```python
from build123d import *

# Parameters (mm, degrees)
SKETCH1_W                    = 79.375
SKETCH1_H                    = 381
BASE_FLANGE1_DEPTH           = 3.175
EDGE_FLANGE1_STRIP_W         = 19.05
EDGE_FLANGE1_STRIP_H         = 3.175
EDGE_FLANGE1_STRIP_CUT_DEPTH = 381
EDGE_FLANGE1_DEPTH           = 381
EDGE_FLANGE2_STRIP_W         = 19.05
EDGE_FLANGE2_STRIP_H         = 3.175
EDGE_FLANGE2_STRIP_CUT_DEPTH = 381
EDGE_FLANGE2_DEPTH           = 381
EDGE_FLANGE3_STRIP_W         = 19.05
EDGE_FLANGE3_STRIP_H         = 3.175
EDGE_FLANGE3_STRIP_CUT_DEPTH = 381
EDGE_FLANGE3_DEPTH           = 381
SKETCH24_W                   = 50.8
SKETCH24_H                   = 31.496
TAB3_DEPTH                   = 3.175
SKETCH27_W                   = 76.2
SKETCH27_H                   = 31.496
TAB4_DEPTH                   = 3.175
SKETCH30_R                   = 1.5875
CUT_EXTRUDE2_DEPTH           = 466.600516135
SKETCH31_R                   = 1.5875
CUT_EXTRUDE3_DEPTH           = 466.600516135


# Sheet-metal steps are written as plain solids
with BuildPart() as part:
    # Sketch1 → Base-Flange1 (new body)
    with BuildSketch(Plane(origin=(0, 0, 0), x_dir=(1, 0, 0), z_dir=(0, 1, 0))):
        with Locations((39.6875, 190.5)):
            Rectangle(SKETCH1_W, SKETCH1_H)
    extrude(amount=-BASE_FLANGE1_DEPTH)

    # Edge-Flange1 strip (across the edge) → Edge-Flange1 strip cut (cut)
    with BuildSketch(Plane.XY.offset(-381)):
        with Locations((-6.35, -1.5875)):
            Rectangle(EDGE_FLANGE1_STRIP_W, EDGE_FLANGE1_STRIP_H)
    extrude(amount=EDGE_FLANGE1_STRIP_CUT_DEPTH, mode=Mode.SUBTRACT)

    # Edge-Flange1 section (across the edge) → Edge-Flange1 (add)
    with BuildSketch(Plane.XY.offset(-381)):
        with BuildLine():
            Line((-3.175, 3.175), (-3.175, 34.925))
            Line((-3.175, 34.925), (0, 34.925))
            Line((0, 34.925), (0, 3.175))
            ThreePointArc((0, 3.175), (0.92993597, 0.92993597), (3.175, 0))
            Line((3.175, 0), (3.175, -3.175))
            ThreePointArc((3.175, -3.175), (-1.315128061, -1.315128061), (-3.175, 3.175))
        make_face()
    extrude(amount=EDGE_FLANGE1_DEPTH)

    # Edge-Flange2 strip (across the edge) → Edge-Flange2 strip cut (cut)
    with BuildSketch(Plane(origin=(0, 34.925, -381), x_dir=(0, -1, 0), z_dir=(0, 0, 1))):
        with Locations((-6.35, -1.5875)):
            Rectangle(EDGE_FLANGE2_STRIP_W, EDGE_FLANGE2_STRIP_H)
    extrude(amount=EDGE_FLANGE2_STRIP_CUT_DEPTH, mode=Mode.SUBTRACT)

    # Edge-Flange2 section (across the edge) → Edge-Flange2 (add)
    with BuildSketch(Plane(origin=(0, 34.925, -381), x_dir=(0, -1, 0), z_dir=(0, 0, 1))):
        with BuildLine():
            Line((-3.175, 3.175), (-3.175, 76.2))
            Line((-3.175, 76.2), (0, 76.2))
            Line((0, 76.2), (0, 3.175))
            ThreePointArc((0, 3.175), (0.92993597, 0.92993597), (3.175, 0))
            Line((3.175, 0), (3.175, -3.175))
            ThreePointArc((3.175, -3.175), (-1.315128061, -1.315128061), (-3.175, 3.175))
        make_face()
    extrude(amount=EDGE_FLANGE2_DEPTH)

    # Edge-Flange3 strip (across the edge) → Edge-Flange3 strip cut (cut)
    with BuildSketch(Plane(origin=(76.2, 34.925, -381), x_dir=(-1, 0, 0), z_dir=(0, 0, 1))):
        with Locations((-6.35, -1.5875)):
            Rectangle(EDGE_FLANGE3_STRIP_W, EDGE_FLANGE3_STRIP_H)
    extrude(amount=EDGE_FLANGE3_STRIP_CUT_DEPTH, mode=Mode.SUBTRACT)

    # Edge-Flange3 section (across the edge) → Edge-Flange3 (add)
    with BuildSketch(Plane(origin=(76.2, 34.925, -381), x_dir=(-1, 0, 0), z_dir=(0, 0, 1))):
        with BuildLine():
            Line((-3.175, 3.175), (-3.175, 34.671))
            Line((-3.175, 34.671), (0, 34.671))
            Line((0, 34.671), (0, 3.175))
            ThreePointArc((0, 3.175), (0.92993597, 0.92993597), (3.175, 0))
            Line((3.175, 0), (3.175, -3.175))
            ThreePointArc((3.175, -3.175), (-1.315128061, -1.315128061), (-3.175, 3.175))
        make_face()
    extrude(amount=EDGE_FLANGE3_DEPTH)

    # Sketch24 → Tab3 (add)
    with BuildSketch(Plane.ZY.offset(-76.2)):
        with Locations((25.4, 16.002)):
            Rectangle(SKETCH24_W, SKETCH24_H)
    extrude(amount=-TAB3_DEPTH)

    # Sketch27 → Tab4 (add)
    with BuildSketch(Plane.ZY.offset(-76.2)):
        with Locations((-419.1, 16.002)):
            Rectangle(SKETCH27_W, SKETCH27_H)
    extrude(amount=-TAB4_DEPTH)

    # Sketch30 → Cut-Extrude2 (cut, through all)
    with BuildSketch(Plane.ZY.offset(-76.2)):
        with Locations(Location((10.16, 25.527, 0), (0, 0, 270))):
            Circle(SKETCH30_R)
        with Locations(Location((41.91, 25.527, 0), (0, 0, 270))):
            Circle(SKETCH30_R)
        with Locations(Location((41.91, 6.477, 0), (0, 0, 270))):
            Circle(SKETCH30_R)
        with Locations(Location((10.16, 6.477, 0), (0, 0, 270))):
            Circle(SKETCH30_R)
    extrude(amount=-CUT_EXTRUDE2_DEPTH, mode=Mode.SUBTRACT)

    # Sketch31 → Cut-Extrude3 (cut, through all)
    with BuildSketch(Plane.ZY.offset(-76.2)):
        with Locations(Location((-447.675, 25.527, 0), (0, 0, 270))):
            Circle(SKETCH31_R)
        with Locations(Location((-447.675, 6.477, 0), (0, 0, 270))):
            Circle(SKETCH31_R)
    extrude(amount=-CUT_EXTRUDE3_DEPTH, mode=Mode.SUBTRACT)


solid = part.part
```
The model under review builds one solid part; all positions refer to its coordinate system, in mm. A direction names the side the tool comes from. Coordinates: 2 decimals unless noted, no trailing zeros. Order: outer loops, then holes, each group sorted by start corner. A loop starts at its lowest first (then second) coordinate and runs counter-clockwise, first axis right, second up. Notation, with made-up numbers: M -33,20 L -16,20 A19 ccw -16,34 Z; hole C 23,25 d9. An arc over 180 degrees is marked long. One line per question, with ' | ' between items.
(1) Insertion check: pin 1 (2.5 mm diameter, centred on x = 78.5, z = -403.5, fed in from +Y); pin 2 (1.9 mm diameter, centred on y = 25.527, z = 10.16, fed in from -X); pin 3 (10 mm diameter, centred on x = 22, y = 3, fed in from +Z). Each pin has a flat end and moves straight along its axis. Give the tip position at first contact, or say it passes through.
Geometry results:
pin 1: stops at y = 31.75 | pin 2: passes through | pin 3: stops at z = 0
(2) The part is to be moulded in two halves that separate along Y. For faces 1 (the face through (-3.175, 17, -193)), 2 (the face through (38, 38.1, -193)), 3 (the face through (41, -3.175, -193)), 4 (the face through (41, 0, -193)), say which applies: +Y half, -Y half, draft (parallel to the pull), parting line (faces both ways), or undercut.
Geometry results:
face 1: draft | face 2: +Y half | face 3: -Y half | face 4: undercut
(3) Add section C-C, the plane z = -225.5. Write out the cut boundary in (x, y) (3 decimals).
Geometry results:
outline: M -3.175,3.175 A6.35 ccw 3.175,-3.175 L 79.375,-3.175 L 79.375,0 L 3.175,0 A3.175 cw 0,3.175 L 0,31.75 A3.175 cw 3.175,34.925 L 73.025,34.925 A3.175 cw 76.2,31.75 L 76.2,0.254 L 79.375,0.254 L 79.375,31.75 A6.35 ccw 73.025,38.1 L 3.175,38.1 A6.35 ccw -3.175,31.75 Z
(4) Machinability: for faces 5 (the face through (0, 18, -193)), 6 (the face through (79.375, 16, -207)), which of the approach directions +Z, -Z, +X, -X, +Y, -Y give a long, thin tool a straight path to every point of the face, cutting with its end or side? Answer none if there is none.
Geometry results:
face 5: +Z, -Z | face 6: +Z, -Z, +X, +Y, -Y
(5) For probe 1 along Y at (x, z) = (53, -266) (3 decimals); probe 2 along X at (y, z) = (22.5, -322) (3 decimals); probe 3 along Y at (x, z) = (77, 10), list the stretches that pass through material, from the lowest coordinate up. Write a range as from..to.
Geometry results:
probe 1: y = -3.175..0, 34.925..38.1 | probe 2: x = -3.175..0, 76.2..79.375 | probe 3: y = 0.25..4.9, 8.06..23.95, 27.11..31.75
(6) Add section A-A, the plane y = 19.5. Write out the cut boundary in (x, z) (3 decimals), then the cut area to 3 significant figures.
Geometry results:
outline: M -3.175,-381 L 0,-381 L 0,0 L -3.175,0 Z; M 76.2,-457.2 L 79.375,-457.2 L 79.375,50.8 L 76.2,50.8 Z | area: 2,820 mm²
(7) Add section B-B, the plane x = 63. Write out the cut boundary in (y, z) (3 decimals).
Geometry results:
outline: M -3.175,-381 L 0,-381 L 0,0 L -3.175,0 Z; M 34.925,-381 L 38.1,-381 L 38.1,0 L 34.925,0 Z
